The model under review builds one solid part; all positions refer to its coordinate system, in mm. A direction names the side the tool comes from. Give positions to 0.01 mm unless a question says otherwise; leave off trailing zeros. Order: outer loops, then holes, each group sorted by start corner. A loop starts at its lowest first (then second) coordinate and runs counter-clockwise, first axis right, second up.
```python
from build123d import *

# Parameters (mm, degrees)
SKETCH1_R           = 11
BOSS_EXTRUDE1_DEPTH = 17
CUT_EXTRUDE1_DEPTH  = 12.5
SKETCH3_R           = 6.5
CUT_EXTRUDE2_DEPTH  = 2
SKETCH4_R           = 3.25
CUT_EXTRUDE3_DEPTH  = 4.5
CHAMFER1_SIZE       = 1.5
CHAMFER2_SIZE       = 0.5


with BuildPart() as part:
    # Sketch1 → Boss-Extrude1 (new body)
    with BuildSketch(Plane.XY):
        Circle(SKETCH1_R)
    extrude(amount=BOSS_EXTRUDE1_DEPTH)

    # Sketch2 → Cut-Extrude1 (cut)
    with BuildSketch(Plane.XY.offset(17)):
        with BuildLine():
            Line((1.6, 2.828869032), (1.6, -2.828869032))
            ThreePointArc((1.6, -2.828869032), (-3.25, 0), (1.6, 2.828869032))
        make_face()
    extrude(amount=-CUT_EXTRUDE1_DEPTH, mode=Mode.SUBTRACT)

    # Sketch3 → Cut-Extrude2 (cut)
    with BuildSketch(Plane.XY.offset(17)):
        Circle(SKETCH3_R)
    extrude(amount=-CUT_EXTRUDE2_DEPTH, mode=Mode.SUBTRACT)

    # Sketch4 → Cut-Extrude3 (cut)
    with BuildSketch(Plane.XY.offset(17)):
        Circle(SKETCH4_R)
    extrude(amount=-CUT_EXTRUDE3_DEPTH, mode=Mode.SUBTRACT)

    # Chamfer1
    chamfer1_edges = [part.edges().sort_by_distance(p)[0] for p in [
        (-11, 0, 0),
    ]]
    chamfer(chamfer1_edges, length=CHAMFER1_SIZE)

    # Chamfer2
    chamfer2_edges = [part.edges().sort_by_distance(p)[0] for p in [
        (-11, 0, 17),
    ]]
    chamfer(chamfer2_edges, length=CHAMFER2_SIZE)


solid = part.part
```
Item 1: Take a section at D-D (z = 3.75). Give the boundary of the cut face in (x, y).
Values found:
outline: circle Ø22 at (0, 0)
Item 2: Draft analysis for pull direction Y (two halves, no side actions). For faces 1 (the flat face through (0, 0, 0)), 2 (the flat face through (1.6, 0, 9)), 3 (the cylindrical face through (-2.38, -10.74, 8.9)), state which applies: released by +Y, released by -Y, zero draft, split by the parting line, or undercut.
Values found:
face 1: zero draft
face 2: undercut
face 3: split by the parting line
Item 3: Take a section at C-C (z = 10.75). Give the boundary of the cut face in (x, y), and give its area (3 significant figures).
Values found:
outline: circle Ø22 at (0, 0); hole (1.6, -2.83) - (1.6, 2.83) arc R3.25 ccw (long way) to start
area: 354 mm2
Item 4: Take a section at B-B (y = 0). Give the boundary of the cut face in (x, z), and give its area (3 significant figures).
Values found:
outline: (-11, 1.5) - (-9.5, 0) - (9.5, 0) - (11, 1.5) - (11, 16.5) - (10.5, 17) - (6.5, 17) - (6.5, 15) - (3.25, 15) - (3.25, 12.5) - (1.6, 12.5) - (1.6, 4.5) - (-3.25, 4.5) - (-3.25, 15) - (-6.5, 15) - (-6.5, 17) - (-10.5, 17) - (-11, 16.5) - close
area: 290 mm2
Item 5: For faces 4 (the flat face through (-2, 3, 15)), 5 (the flat face through (5, 5, 17)), list the 3-axis set-ups (+Z, -Z, +X, -X, +Y, -Y) from which the entire face can be reached by the end or side of a thin tool; tool diameter is ignored.
Values found:
face 4: +Z
face 5: +Z, +X, -X, +Y, -Y
Item 6: Take a section at A-A (x = 0). Give the boundary of the cut face in (y, z), and give its area (3 significant figures).
Values found:
outline: (-11, 1.5) - (-9.5, 0) - (9.5, 0) - (11, 1.5) - (11, 16.5) - (10.5, 17) - (6.5, 17) - (6.5, 15) - (3.25, 15) - (3.25, 4.5) - (-3.25, 4.5) - (-3.25, 15) - (-6.5, 15) - (-6.5, 17) - (-10.5, 17) - (-11, 16.5) - close
area: 277 mm2
Item 7: Clearance check with flat-ended pins moving along their axes: pin 1 Ø8 at (x, z) = (-6.5, 12) entering from -Y; pin 2 Ø10 at (x, z) = (6, 12.5) entering from -Y; pin 3 Ø0.8 at (x, y) = (2, -0.5) entering from +Z. State where each tip first meets the part, or that it passes through.
Values found:
pin 1: stops at y = -10.71
pin 2: stops at y = -10.95
pin 3: stops at z = 12.5
Item 8: For line 1 (Y direction, x = 0, z = 9.75); line 2 (X direction, y = 1.75, z = 14.5); line 3 (Y direction, x = 4.5, z = 16.25), list the stretches that pass through material, from the lowest coordinate up.
Values found:
line 1: y = -11 to -3.25, 3.25 to 11
line 2: x = -10.86 to -2.74, 2.74 to 10.86
line 3: y = -10.04 to -4.69, 4.69 to 10.04
